Source: three-view drawing plus pictorial views. Frame: mm from the lowest corner of the part. A direction names the side the tool comes from. Give positions to 0.01 mm unless a question says otherwise; leave off trailing zeros. Order: outer loops, then holes, each group sorted by start corner. A loop starts at its lowest first (then second) coordinate and runs counter-clockwise, first axis right, second up.
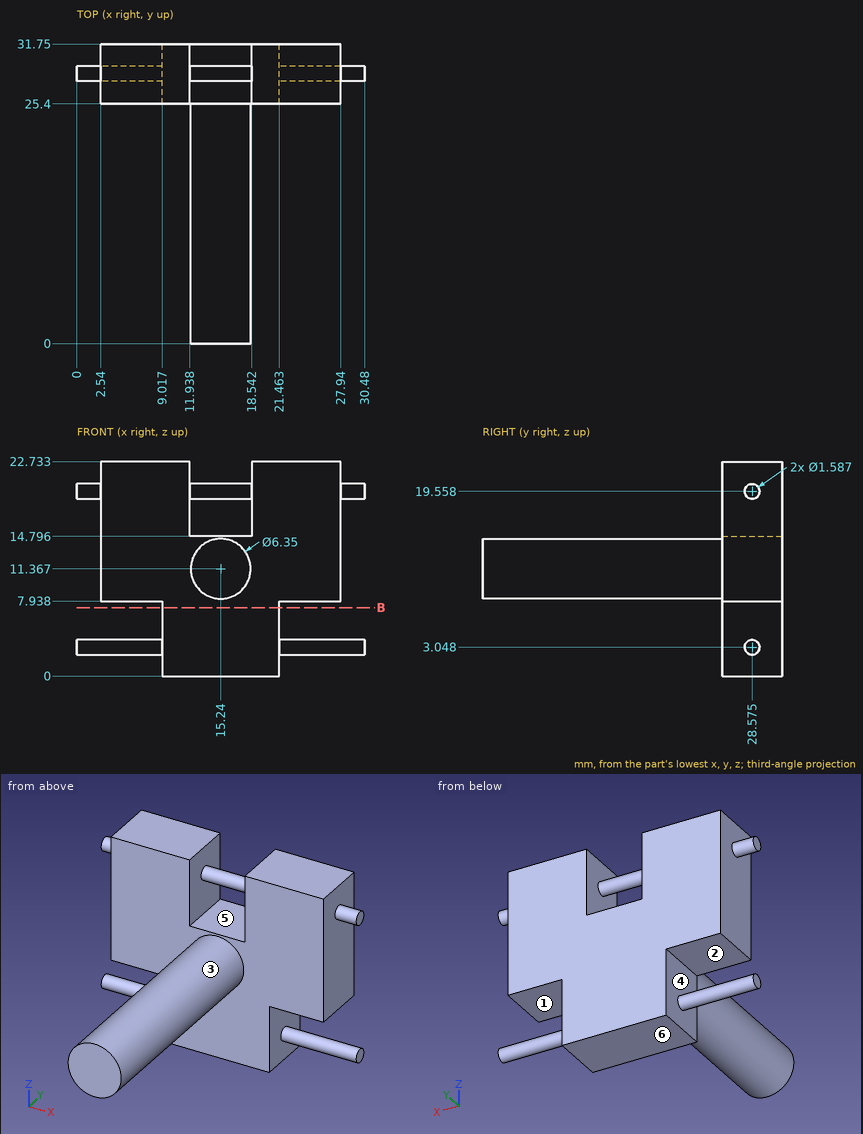
1) Reachability of the marked faces 1, 2 and 3 from +Z, -Z, +X, -X, +Y, -Y: full face, straight path, thin tool, end or side. Return the list, or none.
Checks:
face 1: +X, +Y, -Y
face 2: -X, +Y, -Y
face 3: -Y
2) Pull-direction query (X, two-part tool) for the marked faces 4, 5 and 6; classes: +X half, -X half, draft (parallel to the pull), parting line (faces both ways), or undercut.
Checks:
face 4: -X half
face 5: undercut
face 6: draft
3) Ray query, L1, parallel to Y at x = 19.5, z = 15; L2, parallel to X at y = 26.5, z = 9.5; L3, parallel to Z at x = 15, y = 10. Return the intervals inside material, ascending.
Checks:
L1: y = 25.4 to 31.75
L2: x = 2.54 to 27.94
L3: z = 8.2 to 14.53
4) First-contact query: pin 1 Ø1.9 at (x, y) = (5, 29.5) entering from -Z; pin 2 Ø10 at (x, z) = (23.5, 16) entering from -Y; pin 3 Ø3 at (y, z) = (27.5, 15) entering from +X. Flat tips, straight axial feed; report the tip coordinate or a pass-through.
Checks:
pin 1: stops at z = 2.25
pin 2: stops at y = 25.4
pin 3: stops at x = 27.94
5) Section query B-B on z = 7.25. Output: boundary loops of the cut face in (x, y).
Checks:
outline: (9.02, 25.4) - (21.46, 25.4) - (21.46, 31.75) - (9.02, 31.75) - close
